Here's how the part is built. I have some questions about the finished solid (model axes, mm). A direction names the side the tool comes from. Coordinates: 2 decimals unless noted, no trailing zeros. Write each loop counter-clockwise with the first axis right and the second up, starting at its lowest first coordinate (ties: lowest second). Pieces come first, ordered by that corner, then holes. Notation, with made-up numbers: (-11, 20) -> (9, 20) arc R23 cw to (9, 31) -> close; hole circle Ø1 at (63.25, 17.25). An arc over 180 degrees is marked (long way). Put each result on its own line as item: value.
```python
from build123d import *

# Parameters (mm, degrees)
RHS_C350_AS_100X50X5_0_RHS_C350_1_DEPTH = 677
SKETCH18_R                              = 3.25
CUT_EXTRUDE1_DEPTH                      = 354.846364966
SKETCH19_R                              = 17.1
CUT_EXTRUDE2_DEPTH                      = 10
SKETCH20_R                              = 22.5
CUT_EXTRUDE3_DEPTH                      = 10
SKETCH12_R                              = 2.25
CUT_EXTRUDE4_DEPTH                      = 10
SKETCH21_R                              = 3.25
CUT_EXTRUDE5_DEPTH                      = 346.806665638
SKETCH22_R                              = 3.25
CUT_EXTRUDE6_DEPTH                      = 354.846364966


with BuildPart() as part:
    # Sketch11 → Rhs c350 as 100X50X5.0 RHS C350(1) (new body)
    with BuildSketch(Plane(origin=(0, -338.5, 0), x_dir=(-1, 0, 0), z_dir=(0, 1, 0))):
        with BuildLine():
            Line((-12.5, -50), (12.5, -50))
            ThreePointArc((12.5, -50), (21.338834765, -46.338834765), (25, -37.5))
            Line((25, -37.5), (25, 37.5))
            ThreePointArc((25, 37.5), (21.338834765, 46.338834765), (12.5, 50))
            Line((12.5, 50), (-12.5, 50))
            ThreePointArc((-12.5, 50), (-21.338834765, 46.338834765), (-25, 37.5))
            Line((-25, 37.5), (-25, -37.5))
            ThreePointArc((-25, -37.5), (-21.338834765, -46.338834765), (-12.5, -50))
        make_face()
        with BuildLine():
            Line((-12.5, 45), (12.5, 45))
            ThreePointArc((12.5, 45), (17.803300859, 42.803300859), (20, 37.5))
            Line((20, 37.5), (20, -37.5))
            ThreePointArc((20, -37.5), (17.803300859, -42.803300859), (12.5, -45))
            Line((12.5, -45), (-12.5, -45))
            ThreePointArc((-12.5, -45), (-17.803300859, -42.803300859), (-20, -37.5))
            Line((-20, -37.5), (-20, 37.5))
            ThreePointArc((-20, 37.5), (-17.803300859, 42.803300859), (-12.5, 45))
        make_face(mode=Mode.SUBTRACT)
    extrude(amount=RHS_C350_AS_100X50X5_0_RHS_C350_1_DEPTH)

    # Sketch18 → Cut-Extrude1 (cut, through all)
    with BuildSketch(Plane(origin=(0, 0, -50), x_dir=(-1, 0, 0), z_dir=(0, 0, -1))):
        with Locations((0, 263.5)):
            Circle(SKETCH18_R)
        with Locations((0, 13.5)):
            Circle(SKETCH18_R)
    extrude(amount=-CUT_EXTRUDE1_DEPTH, mode=Mode.SUBTRACT)

    # Sketch19 → Cut-Extrude2 (cut)
    with BuildSketch(Plane(origin=(25, 0, 0), x_dir=(0, 0, -1), z_dir=(1, 0, 0))):
        with Locations(Location((0, 138.5, 0), (0, 0, 90))):
            Circle(SKETCH19_R)
    extrude(amount=-CUT_EXTRUDE2_DEPTH, mode=Mode.SUBTRACT)

    # Sketch20 → Cut-Extrude3 (cut)
    with BuildSketch(Plane.ZY.offset(25)):
        with Locations(Location((0, 138.5, 0), (0, 0, 270))):
            Circle(SKETCH20_R)
    extrude(amount=-CUT_EXTRUDE3_DEPTH, mode=Mode.SUBTRACT)

    # Sketch12 → Cut-Extrude4 (cut)
    with BuildSketch(Plane(origin=(25, 0, 0), x_dir=(0, 0, -1), z_dir=(1, 0, 0))):
        with Locations(Location((14.849242405, 153.349242405, 0), (0, 0, 90))):
            Circle(SKETCH12_R)
        with Locations(Location((-14.849242405, 153.349242405, 0), (0, 0, 90))):
            Circle(SKETCH12_R)
        with Locations(Location((-14.849242405, 123.650757595, 0), (0, 0, 90))):
            Circle(SKETCH12_R)
        with Locations(Location((14.849242405, 123.650757595, 0), (0, 0, 90))):
            Circle(SKETCH12_R)
    extrude(amount=-CUT_EXTRUDE4_DEPTH, mode=Mode.SUBTRACT)

    # Sketch21 → Cut-Extrude5 (cut, through all)
    with BuildSketch(Plane.ZY.offset(25)):
        with Locations(Location((-27.5, -298.5, 0), (0, 0, 270))):
            Circle(SKETCH21_R)
        with Locations(Location((27.5, -298.5, 0), (0, 0, 270))):
            Circle(SKETCH21_R)
    extrude(amount=-CUT_EXTRUDE5_DEPTH, mode=Mode.SUBTRACT)

    # Sketch22 → Cut-Extrude6 (cut, through all)
    with BuildSketch(Plane(origin=(0, 0, -50), x_dir=(-1, 0, 0), z_dir=(0, 0, -1))):
        with Locations((0, -313.5)):
            Circle(SKETCH22_R)
    extrude(amount=-CUT_EXTRUDE6_DEPTH, mode=Mode.SUBTRACT)


solid = part.part
```
Item 1: Please list where these lines run through material, in increasing order: line 1 along Y through (x, z) = (0, -48); line 2 along X through (y, z) = (71.5, -31); line 3 along Z through (x, y) = (7.5, 305). Write a range as from..to.
Output:
line 1: y = -338.5..-316.75, -310.25..10.25, 16.75..260.25, 266.75..338.5
line 2: x = -25..-20, 20..25
line 3: z = -50..-45, 45..50
Item 2: Imagine slicing it at B-B on y = -245.5. Write out the boundary of the cut face in (x, z), then the cut area to 3 significant figures.
Output:
outline: (-25, -37.5) arc R12.5 ccw to (-12.5, -50) -> (12.5, -50) arc R12.5 ccw to (25, -37.5) -> (25, 37.5) arc R12.5 ccw to (12.5, 50) -> (-12.5, 50) arc R12.5 ccw to (-25, 37.5) -> close; hole (-20, -37.5) arc R7.5 ccw to (-12.5, -45) -> (12.5, -45) arc R7.5 ccw to (20, -37.5) -> (20, 37.5) arc R7.5 ccw to (12.5, 45) -> (-12.5, 45) arc R7.5 ccw to (-20, 37.5) -> close
area: 1,310 mm²
Item 3: If we mould it in two halves opening along Z, with no side actions, what happens to faces 4 (the flat face through (-20, -5, 1)), 5 (the cylindrical face through (22.54, 154.81, 5.14)), 6 (the flat face through (0, -5, 50)), 7 (the cylindrical face through (21.435, -4.739, -46.241))? For each: released by +Z, released by -Z, zero draft, split by the parting line, or undercut.
Output:
face 4: undercut
face 5: undercut
face 6: released by +Z
face 7: released by -Z
Item 4: Imagine slicing it at A-A on y = 138.5. Write out the boundary of the cut face in (x, z), then the cut area to 3 significant figures.
Output:
outline: (-25, -37.5) arc R12.5 ccw to (-12.5, -50) -> (12.5, -50) arc R12.5 ccw to (25, -37.5) -> (25, -17.1) -> (20, -17.1) -> (20, -37.5) arc R7.5 cw to (12.5, -45) -> (-12.5, -45) arc R7.5 cw to (-20, -37.5) -> (-20, -22.5) -> (-25, -22.5) -> close; (-25, 22.5) -> (-20, 22.5) -> (-20, 37.5) arc R7.5 cw to (-12.5, 45) -> (12.5, 45) arc R7.5 cw to (20, 37.5) -> (20, 17.1) -> (25, 17.1) -> (25, 37.5) arc R12.5 ccw to (12.5, 50) -> (-12.5, 50) arc R12.5 ccw to (-25, 37.5) -> close
area: 918 mm²
Item 5: Which directions (+Z, -Z, +X, -X, +Y, -Y) give clear straight access to the entire face, cutting with the end or side of a thin tool? Please do faces 1 (the flat face through (20, -5, -1)), 2 (the cylindrical face through (-21.241, -4.739, -46.435)), 3 (the cylindrical face through (-22.535, 117.716, -8.618)).
Output:
face 1: +Y, -Y
face 2: -Z, -X, +Y, -Y
face 3: -X
Item 6: For P1, Ø5, axis at x = 0, y = 13.5, coming from the +Z side; P2, Ø1, axis at x = -19, y = -118, coming from the -Z side, each with a flat end and sliding along its axis, tell me the tip position at first contact or that it passes through.
Output:
P1: passes through
P2: stops at z = -48.47
